Design review of the part built by this model. Coordinates are the model's own, in mm. A direction names the side the tool comes from. Round coordinates to 2 decimals unless told otherwise and drop trailing zeros. Order: outer loops, then holes, each group sorted by start corner. A loop starts at its lowest first (then second) coordinate and runs counter-clockwise, first axis right, second up. Notation, with made-up numbers: M 31,28.5 L 48,28.5 A9 ccw 48,39.5 Z; hole C 55,7.25 d11. An arc over 180 degrees is marked long. Use a Markdown table: item, result. Add a question column.
(1) To check wall thickness, follow probe 1 along X at (y, z) = (0.35, 0); probe 2 along Z at (x, y) = (23.1, 0.65); probe 3 along X at (y, z) = (0.4, 0). State the ranges of each line that lie inside material, in increasing order. Write a range as from..to.
(2) Take a section at A-A (x = 23.1). Write out the cut boundary in (y, z), then the cut area to 3 significant figures.
(3) Take a section at C-C (z = -5). Write out the cut boundary in (x, y).
(4) Take a section at B-B (y = 28). Write out the cut boundary in (x, z), then the cut area to 3 significant figures.
(5) For pin 1 (1.5 mm diameter, centred on y = 43.5, z = 4.5, fed in from +X); pin 2 (4 mm diameter, centred on x = 25.5, z = 1, fed in from -Y); pin 3 (7.5 mm diameter, centred on y = 54.7, z = 0, fed in from +X); pin 4 (3.5 mm diameter, centred on y = 23.1, z = 0, fed in from +X), all flat-tipped, find the tip position at first contact; note any pin that passes through.
(6) The part is to be moulded in two halves that separate along Z. For faces 3 (the face through (32, 2, 0)), 4 (the face through (59.6, 1, 5)), 5 (the face through (0.482, 20.175, 0.384)), say which applies: released by +Z, released by -Z, zero draft, split by the parting line, or undercut.
(7) Machinability: for faces 1 (the face through (2, 33, 0)), 2 (the face through (51.775, 0.482, -0.384)), which of the approach directions +Z, -Z, +X, -X, +Y, -Y give a long, thin tool a straight path to every point of the face, cutting with its end or side? Answer none if there is none.
(8) Take a section at D-D (z = 1.5). Count the separate pieces of the cut face and the enclosed holes in it, then the cut area to 3 significant figures.
```python
from build123d import *

# Parameters (mm, degrees)
BOSS_EXTRU_1_DEPTH                         = 7
CONG_1_R                                   = 7
FRAISAGE_POUR_VIS_T_TE_FRAIS_E_6_2_COUNT   = 2
FRAISAGE_POUR_VIS_T_TE_FRAIS_E_6_2_PITCH   = 31.6
FRAISAGE_POUR_VIS_T_TE_FRAIS_E_6_3_A_COUNT = 2
FRAISAGE_POUR_VIS_T_TE_FRAIS_E_6_3_A_PITCH = 31.6


with BuildPart() as part:
    # Esquisse1 → Boss.-Extru.1 (new, symmetric)
    with BuildSketch(Plane.XY):
        with BuildLine():
            Line((0, 3), (0, 61.7))
            Line((0, 61.7), (2, 61.7))
            Line((2, 61.7), (2, 3))
            ThreePointArc((2, 3), (2.292893219, 2.292893219), (3, 2))
            Line((3, 2), (61.7, 2))
            Line((61.7, 2), (61.7, 0))
            Line((61.7, 0), (3, 0))
            ThreePointArc((3, 0), (0.878679656, 0.878679656), (0, 3))
        make_face()
    extrude(amount=BOSS_EXTRU_1_DEPTH, both=True)

    # Congé1
    cong_1_edges = [part.edges().sort_by_distance(p)[0] for p in [
        (1, 61.7, -7),
        (1, 61.7, 7),
        (61.7, 1, -7),
        (61.7, 1, 7),
    ]]
    fillet(cong_1_edges, radius=CONG_1_R - 0.0001)  # a hair under: the kernel refuses the full size

    # Esquisse2 → Fraisage pour vis _ t_te frais_e _ 6 pan (revolve, cut)
    with BuildSketch(Plane(origin=(54.7, 2, 0), x_dir=(0, 0, 1), z_dir=(1, 0, 0))):
        Polygon((0, 0), (0, 2), (2.95, 2), (2.95, 1.05), (4, 0), align=None)
    fraisage_pour_vis_t_te_frais_e_6_pan = revolve(axis=Axis((54.7, 8.35, 0), (0, -1, 0)), mode=Mode.SUBTRACT)

    # Fraisage pour vis _ t_te frais_e _ 6 2: Fraisage pour vis _ t_te frais_e _ 6 pan ×2
    with Locations(*[(-i * FRAISAGE_POUR_VIS_T_TE_FRAIS_E_6_2_PITCH, 0, 0) for i in range(1, FRAISAGE_POUR_VIS_T_TE_FRAIS_E_6_2_COUNT)]):
        add(fraisage_pour_vis_t_te_frais_e_6_pan, mode=Mode.SUBTRACT)

    # Esquisse4 → Fraisage pour vis _ t_te frais_e _ 6 3 (revolve, cut)
    with BuildSketch(Plane(origin=(2, 54.7, 0), x_dir=(0, 0, -1), z_dir=(0, 1, 0))):
        Polygon((0, 0), (0, 2), (2.95, 2), (2.95, 1.05), (4, 0), align=None)
    fraisage_pour_vis_t_te_frais_e_6_3 = revolve(axis=Axis((8.35, 54.7, 0), (-1, 0, 0)), mode=Mode.SUBTRACT)

    # Fraisage pour vis _ t_te frais_e _ 6 3 a: Fraisage pour vis _ t_te frais_e _ 6 3 ×2
    with Locations(*[(0, -i * FRAISAGE_POUR_VIS_T_TE_FRAIS_E_6_3_A_PITCH, 0) for i in range(1, FRAISAGE_POUR_VIS_T_TE_FRAIS_E_6_3_A_COUNT)]):
        add(fraisage_pour_vis_t_te_frais_e_6_3, mode=Mode.SUBTRACT)


solid = part.part
```
Verdict:
| question | item | result |
|---|---|---|
| 1 | probe 1 | x = 1.59..20.15, 26.05..51.75, 57.65..61.7 |
| 1 | probe 2 | z = -7..-2.95, 2.95..7 |
| 1 | probe 3 | x = 1.5..20.15, 26.05..51.75, 57.65..61.7 |
| 2 | outline | M 0,-7 L 2,-7 L 2,-4 L 0.95,-2.95 L 0,-2.95 Z; M 0,2.95 L 0.95,2.95 L 2,4 L 2,7 L 0,7 Z |
| 2 | area | 15.1 mm^2 |
| 3 | outline | M 0,3 A3 ccw 3,0 L 59.6,0 L 59.6,2 L 3,2 A1 cw 2,3 L 2,59.6 L 0,59.6 Z |
| 4 | outline | M 0,-7 L 2,-7 L 2,7 L 0,7 Z |
| 4 | area | 28.0 mm^2 |
| 5 | pin 1 | stops at x = 2 |
| 5 | pin 2 | stops at y = 0 |
| 5 | pin 3 | stops at x = 1.75 |
| 5 | pin 4 | passes through |
| 6 | face 3 | zero draft |
| 6 | face 4 | released by +Z |
| 6 | face 5 | undercut |
| 7 | face 1 | +Z, -Z, +X, +Y |
| 7 | face 2 | +Y, -Y |
| 8 | separate pieces | 5 |
| 8 | enclosed holes | 0 |
| 8 | area | 195 mm^2 |
